Could you check a few things on this model? Use its own coordinates, in mm. Give positions to 0.01 mm unless a question says otherwise; leave off trailing zeros. Order: outer loops, then holes, each group sorted by start corner. A loop starts at its lowest first (then second) coordinate and runs counter-clockwise, first axis right, second up. Notation, with made-up numbers: M 4,-26 L 45,-26 A13 ccw 45,-18 Z; hole C -28.5,88 d2. An arc over 180 degrees is marked long. Use a Markdown table: item, result. Add a question column.
Item 1: If I drill on L1, parallel to X at y = -3.7, z = -87.5; L2, parallel to Z at x = -50, y = -3.65; L3, parallel to Z at x = 43, y = -3.9, over which ranges is the centre line in solid material (lowest first)? Write a range as from..to.
Item 2: Suppose I cut it at B-B on z = -48. Write out the boundary of the cut face in (x, y).
Item 3: Suppose I cut it at A-A on x = 7.5. Write out the boundary of the cut face in (y, z).
Item 4: I'm going to push flat-ended pins straight in: pin 1 Ø4 at (x, z) = (-50, -18) entering from +Y; pin 2 Ø2.5 at (x, z) = (-7.5, -30) entering from +Y. Where does each tip first touch, or does it pass through?
Item 5: If we mould it in two halves opening along Z, with no side actions, what happens to faces 1 (the face through (-18.07, -2.54, -89.2)), 2 (the face through (-50.07, -2.54, -89.2)), 3 (the face through (1, -2, 0)), 4 (the face through (-56.07, -2.54, -171.5))? For each: released by +Z, released by -Z, zero draft, split by the parting line, or undercut.
Autodesk Inventor part; units mm, degrees
ref_plane "YZ Plane" through (0, 0, 0) normal (1, 0, 0) x (0, 1, 0)
ref_plane "XZ Plane" through (0, 0, 0) normal (0, 1, 0) x (-1, 0, 0)
ref_plane "XY Plane" through (0, 0, 0) normal (0, 0, 1) x (1, 0, 0)
sketch "Sketch1" plane through (0, 0, 0) normal (0, 1, 0) x (-1, 0, 0)
  line L0 (57.5, -173) -> (57.5, -173) construction
  line L1 (-57.5, -173) -> (-57.5, 0) construction
  line L2 (-57.5, 0) -> (57.5, 0)
  line L3 (57.5, 0) -> (57.5, -173) construction
  line L4 (80.5, 0) -> (-80.5, 0) construction
  line L5 (0, -207.6) -> (0, 34.6) construction
  line L6 (57.5, -173) -> (-57.5, -173)
  line L7 (-57.5, -173) -> (-57.5, -173) construction
  line L8 (57.5, 0) -> (-55.1767, 0)
  line L9 (57.5, -40) -> (-57.5, -40) construction
  line L10 (-57.5, -40) -> (-57.5, 0)
  line L11 (-57.5, 0) -> (57.5, 0)
  line L12 (57.5, 0) -> (57.5, -40)
  line L13 (-57.5, -173) -> (-57.5, -40)
  line L14 (57.5, -173) -> (57.5, -40)
  point P0 (0, 0)
  dimension "width" = 115
  dimension "Length" = 173
  dimension "d2" = 115
  dimension "d112" = 40
extrude "Base" add sketch "Sketch1" against normal blind 5
sketch "Sketch11" plane through (0, 0, 0) normal (0, 1, 0) x (1, 0, 0)
  line L0 (0, 207.6) -> (0, -34.6) construction
  line L1 (-57.5, 0) -> (57.5, 0) construction
  line L2 (57.5, 173) -> (-57.5, 173)
  line L3 (-50, 18) -> (50, 18) construction
  line L4 (50, 18) -> (50, 48) construction
  line L5 (50, 48) -> (-50, 48) construction
  line L6 (-50, 48) -> (-50, 18) construction
  point P0 (0, 0)
  point P1 (50, 168)
  point P2 (-50, 168)
  dimension "d91" = 18
  dimension "d92" = 50
  dimension "d93" = 5
  dimension "d94" = 50
  dimension "d113" = 30
hole "Mounting Holes" at (50, 0, -18) at (-50, 0, -18) at (50, 0, -168) at (-50, 0, -168) at (-50, 0, -48) at (50, 0, -48) direction (0, -1, 0) diameter 3.4 depth 6
fillet "Fillet1" radius 5 4 edges at (-57.5, -2.5, 0) (57.5, -2.5, -173) (-57.5, -2.5, -173) (57.5, -2.5, 0)
sketch "Sketch12" plane through (0, 0, 0) normal (0, 1, 0) x (1, 0, 0)
  line L0 (-6, 149) -> (43, 149) construction
  line L1 (43, 149) -> (43, 91) construction
  line L2 (43, 91) -> (-6, 91) construction
  line L3 (-6, 91) -> (-6, 149) construction
  line L4 (-57.5, 168) -> (-57.5, 5)
  line L5 (0, 207.6) -> (0, -34.6)
  line L6 (-52.5, 0) -> (52.5, 0)
  circle A0 centre (-50, 48) radius 1.7
  line L7 (52.5, 173) -> (-52.5, 173)
  circle A1 centre (50, 48) radius 1.7
  circle A2 centre (50, 168) radius 1.7
  point P0 (0, 0)
  point P1 (0, 0)
  point P2 (52.2987, 0)
  point P3 (-57.5, 40)
  point P4 (0, 0)
  dimension "d104" = 58
  dimension "d263" = 24
  dimension "d266" = 49
  dimension "d267" = 7
hole "RasPi Mounting Holes" at (-6, 0, -149) at (43, 0, -149) at (43, 0, -91) at (-6, 0, -91) direction (0, -1, 0) diameter 3.4 depth 6
sketch "Sketch15" plane through (0, 0, 0) normal (0, 1, 0) x (1, 0, 0)
  line L0 (-18, 149) -> (-18, 87.5) construction
  line L1 (-18, 87.5) -> (-50, 87.5) construction
  line L2 (-50, 87.5) -> (-50, 149) construction
  line L3 (-50, 149) -> (-18, 149) construction
  line L4 (-52.5, 0) -> (52.5, 0)
  circle A0 centre (43, 149) radius 1.7
  circle A1 centre (50, 48) radius 1.7
  circle A2 centre (-50, 48) radius 1.7
  point P0 (0, 0)
  point P1 (0, 0)
  dimension "d122" = 32
  dimension "d123" = 61.5
hole "LM2596 Mounting Holes" at (-18, 0, -149) at (-18, 0, -87.5) at (-50, 0, -87.5) at (-50, 0, -149) direction (0, -1, 0) diameter 3.4 depth 6
sketch "Sketch16" plane through (0, 0, 0) normal (0, 1, 0) x (1, 0, 0)
  line L0 (-7.5, 16.5) -> (7.5, 16.5) construction
  line L1 (7.5, 16.5) -> (7.5, 30) construction
  line L2 (7.5, 30) -> (-7.5, 30) construction
  line L3 (-7.5, 30) -> (-7.5, 16.5) construction
  line L4 (52.5, 173) -> (-52.5, 173)
  line L5 (-52.5, 0) -> (52.5, 0)
  point P0 (0, 0)
  point P1 (0, 30)
  point P2 (0, 173)
  dimension "d132" = 15
  dimension "d133" = 13.5
  dimension "d264" = 16.5
hole "Camera Mount Mounting Holes" at (-7.5, 0, -30) at (-7.5, 0, -16.5) at (7.5, 0, -16.5) at (7.5, 0, -30) direction (0, -1, 0) diameter 3.4 depth 6
sketch "Sketch17" plane through (0, 0, 0) normal (0, 1, 0) x (1, 0, 0)
  spline S0 degree 4 poles (20.2958, 49.4851) (20.6789, 48.9084) (23.4396, 47.5095) (25.9197, 47.6138) (27.8901, 48.6422) (29.1867, 50.3145) (29.4114, 52.1793) (28.5047, 55.2295) (25.5201, 55.758) (20.7186, 56.8474) (23.8724, 60.2591) (26.3838, 58.5227) (28.1257, 57.2645) knots 0 0 0 0 0 0.20272 0.281354 0.355201 0.433006 0.519581 0.610324 0.697239 0.780232 1 1 1 1 1
  line L0 (28.1257, 57.2645) -> (29.7111, 59.2874)
  line L1 (20.2958, 49.4851) -> (21.6797, 51.6642)
  spline S1 degree 4 poles (21.6797, 51.6642) (22.294, 51.399) (22.8002, 50.5746) (25.5673, 49.8354) (26.8617, 51.423) (26.2496, 52.8197) (24.0458, 53.1534) (23.329, 53.4897) (21.3928, 54.1292) (20.3004, 55.4262) (19.7305, 56.5102) (20.0555, 59.7919) (23.1279, 61.9518) (27.765, 61.4454) (29.2944, 59.5103) (29.7111, 59.2874) knots 0 0 0 0 0 0.144957 0.205265 0.266901 0.324627 0.385746 0.449033 0.50901 0.575778 0.647334 0.728378 0.816759 1 1 1 1 1
  line L2 (19.0392, 48.0812) -> (19.0392, 61.1238)
  line L3 (19.0392, 61.1238) -> (16.3103, 61.1165)
  line L4 (16.3103, 61.1165) -> (16.3103, 57.2645)
  line L5 (16.3005, 50.6209) -> (16.3005, 54.6823)
  line L6 (16.3005, 54.6823) -> (13.9834, 54.6823)
  line L7 (16.3005, 50.6209) -> (13.9834, 50.6209)
  line L8 (19.0392, 48.0812) -> (13.9055, 48.0812)
  line L9 (16.3103, 57.2645) -> (13.9055, 57.2645)
  spline S2 degree 4 poles (13.9055, 48.0812) (12.4376, 47.8656) (9.7169, 48.6839) (8.992, 53.4734) (10.0175, 55.7505) (11.813, 57.33) (13.9055, 57.2645) knots 0 0 0 0 0 0.424255 0.584368 1 1 1 1 1
  spline S3 degree 4 poles (13.9834, 50.6209) (12.4963, 50.3877) (10.9812, 52.4197) (12.1533, 54.6228) (13.9834, 54.6823) knots 0 0 0 0 0 1 1 1 1 1
  line L10 (5.611, 51.8606) -> (5.611, 61.1378)
  line L11 (5.611, 61.1378) -> (2.2951, 61.1378)
  line L12 (2.2951, 61.1378) -> (2.2951, 60.9623)
  line L13 (2.2951, 60.9623) -> (2.2951, 57.2161)
  line L14 (2.2951, 57.2161) -> (0.5839, 57.2161)
  line L15 (0.5839, 57.2161) -> (-1.936, 61.1378)
  line L16 (-1.936, 61.1378) -> (-5.9376, 61.1378)
  line L17 (-5.9376, 61.1378) -> (-3.4177, 57.2161)
  line L18 (5.611, 51.8606) -> (2.2951, 51.8606)
  line L19 (2.2951, 51.8606) -> (2.2951, 53.8306)
  line L20 (2.2951, 53.8306) -> (-1.6405, 53.8306)
  line L21 (-1.6405, 53.8306) -> (-1.6405, 51.2415)
  line L22 (-1.6405, 51.2415) -> (5.611, 51.2415)
  line L23 (5.611, 51.2415) -> (5.611, 47.9336)
  line L24 (5.611, 47.9336) -> (-3.7057, 47.9336)
  line L25 (-5.0121, 49.3829) -> (-5.0121, 55.5531)
  arc A0 (-3.4177, 57.2161) -> (-5.0121, 55.5531) centre (-3.281, 55.4892) ccw
  arc A1 (-5.0121, 49.3829) -> (-3.7057, 47.9336) centre (-2.6718, 50.1788) ccw
  line L26 (-6.9039, 47.9336) -> (-10.2687, 47.9336)
  line L27 (-10.2687, 47.9336) -> (-10.2687, 61.1378)
  line L28 (-10.2687, 61.1378) -> (-6.9039, 61.1378)
  line L29 (-6.9039, 61.1378) -> (-6.9039, 47.9336)
  line L30 (-11.8026, 47.9336) -> (-11.8026, 51.2415)
  line L31 (-11.8026, 51.2415) -> (-15.1713, 51.2415)
  line L32 (-15.1713, 51.2415) -> (-15.1713, 61.1378)
  line L33 (-15.1713, 61.1378) -> (-18.4823, 61.1378)
  line L34 (-18.4823, 61.1378) -> (-18.4823, 47.9336)
  line L35 (-18.4823, 47.9336) -> (-11.8026, 47.9336)
  line L36 (-19.0962, 47.9336) -> (-19.0962, 51.2415)
  line L37 (-19.0962, 51.2415) -> (-21.5406, 51.2415)
  line L38 (-21.5406, 51.2415) -> (-23.787, 47.9336)
  line L39 (-23.787, 47.9336) -> (-19.0962, 47.9336)
  line L40 (-24.4617, 47.9274) -> (-24.4617, 61.1378)
  line L41 (-24.4617, 61.1378) -> (-27.7836, 61.1378)
  line L42 (-27.7836, 61.1378) -> (-27.7836, 47.9274)
  line L43 (-27.7836, 47.9274) -> (-24.4617, 47.9274)
  line L44 (-28.3589, 52.8456) -> (-28.3589, 56.1975)
  line L45 (-28.3589, 56.1975) -> (-30.851, 56.1975)
  line L46 (-30.851, 52.8456) -> (-28.3589, 52.8456)
  line L47 (-27.7836, 47.9274) -> (-27.7836, 51.2654)
  line L48 (-27.7836, 51.2654) -> (-32.8922, 51.2654)
  line L49 (-32.8922, 47.9274) -> (-27.7836, 47.9274)
  line L50 (-32.8922, 47.9274) -> (-35.0606, 51.2654)
  line L51 (-35.0606, 51.2654) -> (-32.8922, 51.2654)
  line L52 (-30.851, 52.8456) -> (-33.0635, 52.8734)
  line L53 (-33.0635, 52.8734) -> (-30.851, 56.1975)
  line L54 (-27.7836, 57.7985) -> (-35.0607, 57.7985)
  line L55 (-35.0607, 57.7985) -> (-32.8922, 61.1378)
  line L56 (-32.8922, 61.1378) -> (-27.7836, 61.1378)
  point P0 (21.8312, 48.4826)
  point P1 (24.6762, 47.7793)
  point P2 (27.8239, 48.7935)
  point P3 (29.2122, 52.0376)
  point P4 (25.048, 55.8974)
  point P5 (22.697, 57.0989)
  point P6 (22.9251, 58.2765)
  point P7 (24.696, 58.9116)
  point P8 (28.2025, 54.5742)
  point P9 (28.8947, 50.19)
  point P10 (26.5311, 48.0478)
  point P11 (22.4682, 51.1588)
  point P12 (23.9337, 50.486)
  point P13 (25.8462, 50.5785)
  point P14 (26.5371, 51.481)
  point P15 (26.0534, 52.5205)
  point P16 (24.2764, 53.1685)
  point P17 (23.1794, 53.5189)
  point P18 (21.5574, 54.2619)
  point P19 (20.447, 55.336)
  point P20 (19.9671, 56.4765)
  point P21 (20.2871, 59.0572)
  point P22 (22.4689, 61.0346)
  point P23 (26.4542, 61.133)
  point P24 (29.0183, 59.8364)
  point P25 (11.4209, 48.5556)
  point P26 (9.7808, 50.5107)
  point P27 (9.4544, 53.0399)
  point P28 (9.8764, 54.8382)
  point P29 (11.0351, 56.3298)
  point P30 (12.7053, 51.0405)
  point P31 (12.0378, 52.3742)
  point P32 (12.4432, 53.8804)
  point P33 (-27.7836, 51.2654)
  point P34 (-3.281, 55.4892)
extrude "SP RITE Logo" [suppressed]
sketch "Sketch18" plane through (0, 0, 0) normal (0, 1, 0) x (1, 0, 0)
  circle A0 centre (-50, 48) radius 1.7
  line L0 (-57.5, 168) -> (-57.5, 5)
  line L1 (-16.9, 35.8) -> (-16.9, 47)
  line L2 (-16.9, 47) -> (-16.9, 60.2)
  point P0 (0, 0)
  dimension "d281" = 40.6
  dimension "d282" = 12.2
  dimension "d284" = 12.2
  dimension "d285" = 33.1
hole "Button Board Mounting Holes" at (-16.9, 0, -60.2) at (-16.9, 0, -35.8) direction (0, -1, 0) diameter 3 end through all
equation "\"d2\" = width"
equation "\"d95\" = HoleDia"
equation "\"d105\" = HoleDia"
equation "\"d125\" = HoleDia"
equation "\"d135\" = HoleDia"
equation "\"HoleDia\" = 3.4"
properties part number "top plate"
Findings below:
| question | item | result |
|---|---|---|
| 1 | L1 | x = -57.5..-51.7, -48.3..-19.7, -16.3..57.5 |
| 1 | L2 | z = -173..-169.7, -166.3..-150.7, -147.3..-89.2, -85.8..-49.7, -46.3..-19.7, -16.3..0 |
| 1 | L3 | z = -173..-150.7, -147.3..-92.7, -89.3..0 |
| 2 | outline | M -57.5,-5 L -51.7,-5 L -51.7,0 L -57.5,0 Z; M -48.3,-5 L 48.3,-5 L 48.3,0 L -48.3,0 Z; M 51.7,-5 L 57.5,-5 L 57.5,0 L 51.7,0 Z |
| 3 | outline | M -5,-173 L 0,-173 L 0,-31.7 L -5,-31.7 Z; M -5,-28.3 L 0,-28.3 L 0,-18.2 L -5,-18.2 Z; M -5,-14.8 L 0,-14.8 L 0,0 L -5,0 Z |
| 4 | pin 1 | stops at y = 0 |
| 4 | pin 2 | passes through |
| 5 | face 1 | undercut |
| 5 | face 2 | undercut |
| 5 | face 3 | released by +Z |
| 5 | face 4 | released by -Z |
